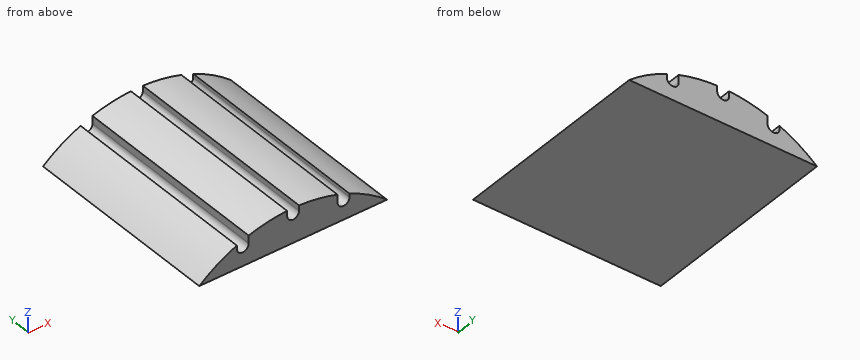
from build123d import *

# Parameters (mm, degrees)
F1_DEPTH = 101.6


with BuildPart() as f1:
    # F0 (on Front) → F1 (new body)
    with BuildSketch(Plane.XZ):
        with BuildLine():
            Line((-47.3245013075, 56.1975), (47.3245013075, 56.1975))
            ThreePointArc((47.3245013075, 56.1975), (38.3009648813, 62.6961204495), (28.4, 67.7584491429))
            Line((28.4, 67.7584491429), (28.4, 66.0049502102))
            ThreePointArc((28.4, 66.0049502102), (25.2876310607, 63.0070554119), (22.4084178523, 66.2295303826))
            Line((22.4084178523, 66.2295303826), (22.4084178523, 69.9687804639))
            ThreePointArc((22.4084178523, 69.9687804639), (12.8187011015, 72.3425762074), (2.997208132, 73.408338584))
            Line((2.997208132, 73.408338584), (2.997208132, 70.7234999449))
            ThreePointArc((2.997208132, 70.7234999449), (-0.002791868, 67.7234999449), (-3.002791868, 70.7234999449))
            Line((-3.002791868, 70.7234999449), (-3.0169040135, 70.7234999449))
            Line((-3.0169040135, 70.7234999449), (-3.0169040135, 73.407531769))
            ThreePointArc((-3.0169040135, 73.407531769), (-12.8301586499, 72.3405450579), (-22.4118081837, 69.9676945753))
            Line((-22.4118081837, 69.9676945753), (-22.4118081837, 66.2708631072))
            ThreePointArc((-22.4118081837, 66.2708631072), (-22.4029534998, 66.1380376833), (-22.4, 66.0049502102))
            ThreePointArc((-22.4, 66.0049502102), (-25.4, 63.0049502102), (-28.4, 66.0049502102))
            Line((-28.4, 66.0049502102), (-28.4, 67.7584491429))
            ThreePointArc((-28.4, 67.7584491429), (-38.3009648813, 62.6961204495), (-47.3245013075, 56.1975))
        make_face()
    extrude(amount=F1_DEPTH)


solid = f1.part
Build history of the part. All positions in model axes, mm. Coordinates: 2 decimals unless noted, no trailing zeros. Order: outer loops, then holes, each group sorted by start corner. A loop starts at its lowest first (then second) coordinate and runs counter-clockwise, first axis right, second up. Notation, with made-up numbers: (-22.75, -32) - (-2.75, -32) arc R9 cw to (-2.75, -22) - close; hole circle Ø2 at (36, 23.5). An arc over 180 degrees is marked (long way). Write each question's results on one line, items separated by ' | '. Start each with the question number.
Item 1: Band-saw the part on C-C on z = 61.5. Write the cut outline in (x, y).
Item 2: Wall check: probe 1 along X at (y, z) = (-78.5, 64.25); probe 2 along X at (y, z) = (-40, 65.25); probe 3 along X at (y, z) = (-48, 69.25). Give the ranges that are in metal, low to high. Write a range as [from, to].
Item 3: Flat gauge pins, fed straight in: pin 1 (1.9 mm diameter, centred on y = -28.5, z = 67.5, fed in from +X); pin 2 (1.1 mm diameter, centred on y = -71, z = 68, fed in from -X) (3 decimals); pin 3 (8 mm diameter, centred on y = -28, z = 69.5, fed in from -X). Where does each tip first touch, or does it go through?
Item 4: Band-saw the part on B-B on x = -25.4. Write the cut outline in (y, z), and give its area (3 significant figures).
Numbers:
1) outline: (-40.19, -101.6) - (40.19, -101.6) - (40.19, 0) - (-40.19, 0) - close
2) probe 1: [-35.63, -27.83], [-22.97, 22.97], [27.83, 35.63] | probe 2: [-33.77, -28.3], [-22.5, 22.5], [28.3, 33.77] | probe 3: [-22.41, -2.62], [2.61, 22.41]
3) pin 1: x = 31.13 | pin 2: x = -29.125 | pin 3: x = -33.28
4) outline: (-101.6, 56.2) - (0, 56.2) - (0, 63) - (-101.6, 63) - close | area: 692 mm^2
